Here's how the part is built. I have some questions about the finished solid (model axes, mm). Give positions to 0.01 mm unless a question says otherwise; leave off trailing zeros. Use a Markdown table: item, result.
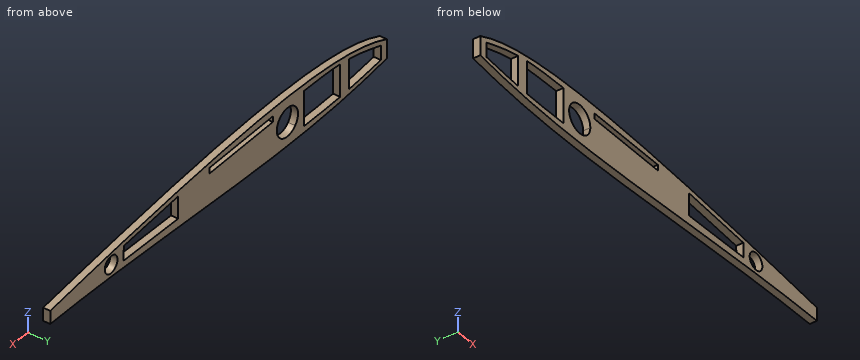
from build123d import *

# Parameters (mm, degrees)
F2_DEPTH = 2.5
F1_R     = 3
F3_DEPTH = 2.5
F5_DEPTH = 2.5
F4_W     = 30
F4_H     = 2
F6_DEPTH = 2.5
F7_DEPTH = 2.5


with BuildPart() as f2:
    # F0 (on Front) → F2 (new body)
    with BuildSketch(Plane.XZ):
        with BuildLine():
            add(Edge.make_bspline(
                [(-96.9805282175, -0.8100506688), (-84.7869920978, 5.1468541776), (-38.6381415733, 10.9636146396), (42.6881882799, 2.4723259958), (100, -4.047003109)],
                knots=[0, 0, 0, 0, 0.374886421, 1, 1, 1, 1], degree=3))
            add(Edge.make_bspline(
                [(-97.5447368223, -7.1186651935), (-99.939251346, -6.5508492693), (-102.885147974, -5.168950634), (-100.0067471137, -2.3789404522), (-96.9805282175, -0.8100506688)],
                knots=[0.0564585679, 0.0564585679, 0.0564585679, 0.0564585679, 0.4847104148, 1, 1, 1, 1], degree=3))
            add(Edge.make_bspline(
                [(-96.5428845142, -7.3406707446), (-96.8949965543, -7.2673488468), (-97.22905608, -7.1935231869), (-97.5447368223, -7.1186651935)],
                knots=[0, 0, 0, 0, 0.0564585679, 0.0564585679, 0.0564585679, 0.0564585679], degree=3))
            add(Edge.make_bspline(
                [(-96.5428845142, -7.3406707446), (-80.7020161693, -9.4302402111), (-44.2471235075, -11.1181020976), (41.8622965332, -3.5518856086), (82.0915186506, -4.6802794425), (100, -4.047003109)],
                knots=[0, 0, 0, 0, 0.2987594418, 0.6837410955, 1, 1, 1, 1], degree=3))
        make_face()
        with BuildLine():
            add(Edge.make_bspline(
                [(-99.8196757147, -4.047003109), (-99.3821638101, -3.2227137691), (-97.9006497107, -2.3042858417), (-96.3385477662, -1.6362179573)],
                knots=[0.5425000514, 0.5425000514, 0.5425000514, 0.5425000514, 1, 1, 1, 1], degree=3))
            add(Edge.make_bspline(
                [(-96.3385477662, -1.6362179573), (-85.7442874691, 3.2900694446), (-38.7960585931, 10.0747672146), (36.943279708, 1.696590452), (86.094097513, -3.3751911245)],
                knots=[0, 0, 0, 0, 0.384923117, 1, 1, 1, 1], degree=3))
            add(Edge.make_bspline(
                [(-97.3825784566, -6.0471531808), (-82.3468325761, -8.841713568), (-44.2551066449, -8.6286827794), (40.9195716837, -3.3120714751), (72.7341022162, -3.1550192186), (86.094097513, -3.3751911245)],
                knots=[0, 0, 0, 0, 0.3131273629, 0.7122131732, 1, 1, 1, 1], degree=3))
            add(Edge.make_bspline(
                [(-97.3825784566, -6.0471531808), (-98.6588937786, -5.8946130057), (-100.1661659123, -5.1778479876), (-99.9138553768, -4.2244412327), (-99.8196757147, -4.047003109)],
                knots=[0, 0, 0, 0, 0.4440177242, 0.5425000514, 0.5425000514, 0.5425000514, 0.5425000514], degree=3))
        make_face(mode=Mode.SUBTRACT)
        with BuildLine():
            add(Edge.make_bspline(
                [(-96.3385477662, -1.6362179573), (-85.7442874691, 3.2900694446), (-38.7960585931, 10.0747672146), (36.943279708, 1.696590452), (86.094097513, -3.3751911245)],
                knots=[0, 0, 0, 0, 0.384923117, 1, 1, 1, 1], degree=3))
            add(Edge.make_bspline(
                [(-99.8196757147, -4.047003109), (-99.3821638101, -3.2227137691), (-97.9006497107, -2.3042858417), (-96.3385477662, -1.6362179573)],
                knots=[0.5425000514, 0.5425000514, 0.5425000514, 0.5425000514, 1, 1, 1, 1], degree=3))
            add(Edge.make_bspline(
                [(-97.3825784566, -6.0471531808), (-98.6588937786, -5.8946130057), (-100.1661659123, -5.1778479876), (-99.9138553768, -4.2244412327), (-99.8196757147, -4.047003109)],
                knots=[0, 0, 0, 0, 0.4440177242, 0.5425000514, 0.5425000514, 0.5425000514, 0.5425000514], degree=3))
            add(Edge.make_bspline(
                [(-97.3825784566, -6.0471531808), (-82.3468325761, -8.841713568), (-44.2551066449, -8.6286827794), (40.9195716837, -3.3120714751), (72.7341022162, -3.1550192186), (86.094097513, -3.3751911245)],
                knots=[0, 0, 0, 0, 0.3131273629, 0.7122131732, 1, 1, 1, 1], degree=3))
        make_face()
        with BuildLine():
            add(Edge.make_bspline(
                [(-96.5428845142, -7.3406707446), (-96.8949965543, -7.2673488468), (-97.22905608, -7.1935231869), (-97.5447368223, -7.1186651935)],
                knots=[0, 0, 0, 0, 0.0564585679, 0.0564585679, 0.0564585679, 0.0564585679], degree=3))
            ThreePointArc((-97.5447368223, -7.1186651935), (-97.052492706, -7.2688477084), (-96.5428845142, -7.3406707446))
        make_face()
    extrude(amount=F2_DEPTH)


with BuildPart() as f2b:
    # F1 (on Front) → F2, piece 2 (new body)
    with BuildSketch(Plane.XZ):
        with Locations((33.7789729238, -1.0305350879)):
            Circle(F1_R)
    extrude(amount=F2_DEPTH)


with BuildPart() as f2c:
    # F1 (on Front) → F2, piece 3 (new body)
    with BuildSketch(Plane.XZ):
        with BuildLine():
            ThreePointArc((-44.542362095, -1.3708024857), (-51.3662704709, 3.2846629299), (-53.2117053896, -4.7672594318))
            Line((-53.2117053896, -4.7672594318), (-45.8404576082, -4.7317403266))
            ThreePointArc((-45.8404576082, -4.7317403266), (-44.8781621403, -3.1722571154), (-44.542362095, -1.3708024857))
        make_face()
        with BuildLine():
            Line((-45.8404576082, -4.7317403266), (-53.2117053896, -4.7672594318))
            ThreePointArc((-53.2117053896, -4.7672594318), (-49.5182693675, -6.3707444394), (-45.8404576082, -4.7317403266))
        make_face()
    extrude(amount=F2_DEPTH)


with BuildPart() as f3_tool:
    # F1 (on Front) → F3 (new body)
    with BuildSketch(Plane.XZ):
        with BuildLine():
            ThreePointArc((-44.542362095, -1.3708024857), (-51.3662704709, 3.2846629299), (-53.2117053896, -4.7672594318))
            Line((-53.2117053896, -4.7672594318), (-45.8404576082, -4.7317403266))
            ThreePointArc((-45.8404576082, -4.7317403266), (-44.8781621403, -3.1722571154), (-44.542362095, -1.3708024857))
        make_face()
        with BuildLine():
            Line((-45.8404576082, -4.7317403266), (-53.2117053896, -4.7672594318))
            ThreePointArc((-53.2117053896, -4.7672594318), (-49.5182693675, -6.3707444394), (-45.8404576082, -4.7317403266))
        make_face()
        with Locations((33.7789729238, -1.0305350879)):
            Circle(F1_R)
    extrude(amount=F3_DEPTH)


with BuildPart() as f2_1:
    add(f2.part)

    # F3: cut by f3_tool
    add(f3_tool.part, mode=Mode.SUBTRACT)

    # F4 (on face) → F5 (cut)
    with BuildSketch(Plane.XZ.offset(2.5)):
        with BuildLine():
            Line((-96.5428845142, -7.3406707446), (-96.5428845142, -0.5989118026))
            add(Edge.make_bspline(
                [(-96.9805282175, -0.8100506688), (-96.8353706427, -0.7391368787), (-96.6894893165, -0.6687582494), (-96.5428845142, -0.5989118026)],
                knots=[0, 0, 0, 0, 0.0044628238, 0.0044628238, 0.0044628238, 0.0044628238], degree=3))
            add(Edge.make_bspline(
                [(-96.9805282175, -0.8100506688), (-100.0067471137, -2.3789404522), (-102.885147974, -5.168950634), (-99.939251346, -6.5508492693), (-97.5447368223, -7.1186651935)],
                knots=[0.0564585679, 0.0564585679, 0.0564585679, 0.0564585679, 0.5717481532, 1, 1, 1, 1], degree=3))
            ThreePointArc((-97.5447368223, -7.1186651935), (-97.052492706, -7.2688477084), (-96.5428845142, -7.3406707446))
        make_face()
    extrude(amount=-F5_DEPTH, mode=Mode.SUBTRACT)

    # F4 (on face) → F6 (cut)
    with BuildSketch(Plane.XZ.offset(2.5)):
        with BuildLine():
            Line((-78.6215588156, -7.3670944992), (-78.6215588156, 3.2958948603))
            add(Edge.make_bspline(
                [(-78.6215588156, 3.2958948603), (-83.9345486349, 2.2532028855), (-88.8194569144, 0.5548157735), (-93.7043651938, -1.1435713386)],
                knots=[0.554896308, 0.554896308, 0.554896308, 0.554896308, 1, 1, 1, 1], degree=3))
            Line((-93.7043651938, -1.1435713386), (-93.7043651938, -6.1954581179))
            add(Edge.make_bspline(
                [(-78.6215588156, -7.3670944992), (-83.7013643272, -7.1077100258), (-88.7028647605, -6.6515840718), (-93.7043651938, -6.1954581179)],
                knots=[0.5793594661, 0.5793594661, 0.5793594661, 0.5793594661, 1, 1, 1, 1], degree=3))
        make_face()
        with BuildLine():
            Line((-57.251535356, -7.4831936508), (-57.251535356, 4.8988820054))
            add(Edge.make_bspline(
                [(-57.251535356, 4.8988820054), (-63.1249518816, 4.7812850577), (-68.9983684072, 4.66368811), (-74.4892291338, 3.9601280834)],
                knots=[0, 0, 0, 0, 0.4418705618, 0.4418705618, 0.4418705618, 0.4418705618], degree=3))
            Line((-74.4892291338, 3.9601280834), (-74.4892291338, -7.5306241193))
            add(Edge.make_bspline(
                [(-57.251535356, -7.4831936508), (-63.0319736557, -7.5857864832), (-68.8124119553, -7.6883793156), (-74.4892291338, -7.5306241193)],
                knots=[0, 0, 0, 0, 0.4658094847, 0.4658094847, 0.4658094847, 0.4658094847], degree=3))
        make_face()
        with Locations((-27.6331795752, 3.8601249214)):
            Rectangle(F4_W, F4_H)
        Polygon((27.7735989974, 1.9125135442), (2.0833725575, 3.8092588075), (2.0833725575, -4.047003109), (27.937149629, -3.2237600535), align=None)
    extrude(amount=-F6_DEPTH, mode=Mode.SUBTRACT)

    # F4 (on face) → F7 (cut)
    with BuildSketch(Plane.XZ.offset(2.5)):
        with BuildLine():
            add(Edge.make_bspline(
                [(62.5460875734, 0.1020588345), (74.6514883615, -1.1873862537), (87.1633646635, -2.586811085), (100, -4.047003109)],
                knots=[0.8599877614, 0.8599877614, 0.8599877614, 0.8599877614, 1, 1, 1, 1], degree=3))
            Line((62.5460875734, 0.1020588345), (62.5460875734, -4.518638291))
            add(Edge.make_bspline(
                [(62.5460875734, -4.518638291), (75.9097127299, -4.3829595873), (88.0075171585, -4.4710790211), (100, -4.047003109)],
                knots=[0.7882160183, 0.7882160183, 0.7882160183, 0.7882160183, 1, 1, 1, 1], degree=3))
        make_face()
    extrude(amount=-F7_DEPTH, mode=Mode.SUBTRACT)


with BuildPart() as f2b_1:
    add(f2b.part)

    # F3: cut by f3_tool
    add(f3_tool.part, mode=Mode.SUBTRACT)


with BuildPart() as f2c_1:
    add(f2c.part)

    # F3: cut by f3_tool
    add(f3_tool.part, mode=Mode.SUBTRACT)


solid = f2_1.part
(1) Will these pins go through, and if not, where does the flat tip stop? pin 1 (0.8 mm diameter, centred on x = -26, y = -1.5, fed in from +Z); pin 2 (1.5 mm diameter, centred on x = 27.5, y = -2, fed in from +Z); pin 3 (6 mm diameter, centred on x = -49.54, z = -1.37, fed in from -Y); pin 4 (7 mm diameter, centred on x = 33.78, z = -1.03, fed in from +Y).
A:
| item | result |
|---|---|
| pin 1 | z = 7.22 |
| pin 2 | z = 3.66 |
| pin 3 | through |
| pin 4 | y = 0 |
(2) If I drill on line 1 (X direction, y = -0.95, z = -1.75); line 2 (X direction, y = -1.05, z = -1.25); line 3 (Z direction, x = -37.5, y = -0.6), over which ranges is the centre line in solid material (lowest first)?
A:
| item | result |
|---|---|
| line 1 | -96.54 to -93.7, -78.62 to -74.49, -57.25 to -54.53, -44.56 to 2.08, 27.89 to 30.87, 36.69 to 62.55 |
| line 2 | -96.54 to -93.7, -78.62 to -74.49, -57.25 to -54.54, -44.54 to 2.08, 27.87 to 30.79, 36.77 to 62.55 |
| line 3 | -9.35 to 2.86, 4.86 to 7.48 |
(3) Suppose I cut it at A-A on y = -1.3. Count the separate pieces of the cut face and the enclosed holes in it, plus the area to 3 significant figures.
A:
| item | result |
|---|---|
| separate pieces | 1 |
| enclosed holes | 6 |
| area | 1,320 mm2 |
